Geometry check sheet. Reference: the model listing, model coordinates, mm. A direction names the side the tool comes from. Coordinates: 2 decimals unless noted, no trailing zeros. Write each loop counter-clockwise with the first axis right and the second up, starting at its lowest first coordinate (ties: lowest second). Pieces come first, ordered by that corner, then holes. Notation, with made-up numbers: (43, 47.25) -> (56, 47.25) arc R22 ccw to (56, 53.25) -> close; hole circle Ø6 at (-31, -38). An arc over 180 degrees is marked (long way). Use a Markdown table: item, result.
Autodesk Inventor part; units mm, degrees
ref_plane "YZ Plane" through (0, 0, 0) normal (1, 0, 0) x (0, 1, 0)
ref_plane "XZ Plane" through (0, 0, 0) normal (0, 1, 0) x (-1, 0, 0)
ref_plane "XY Plane" through (0, 0, 0) normal (0, 0, 1) x (1, 0, 0)
sketch "Sketch1" plane through (0, 0, 0) normal (1, 0, 0) x (0, 1, 0)
  line L0 (0, 0) -> (-25.4, 0)
  line L1 (-25.4, 0) -> (-25.4, -25.4)
  line L2 (-25.4, -25.4) -> (0, -25.4)
  line L3 (0, -25.4) -> (0, 0)
  line L4 (-3.175, -22.225) -> (-22.225, -22.225)
  line L5 (-22.225, -22.225) -> (-22.225, -3.175)
  line L6 (-22.225, -3.175) -> (-3.175, -3.175)
  line L7 (-3.175, -3.175) -> (-3.175, -22.225)
  dimension "d0" = 25.4
  dimension "d1" = 25.4
  dimension "d2" = 3.175
extrude "Extrusion1" add sketch "Sketch1" along normal blind 476.25
sketch "Sketch2" plane through (0, 0, 0) normal (0, 1, 0) x (1, 0, 0)
  line L0 (0, 3.175) -> (0, 22.225)
  line L1 (0, 12.7) -> (476.25, 12.7) construction
  line L2 (0, 25.4) -> (476.25, 25.4)
  line L3 (476.25, 25.4) -> (476.25, 0)
  point P0 (0, 0)
  point P1 (438.15, 12.7)
  point P2 (12.7, 12.7)
  point P3 (38.1, 12.7)
  point P4 (459.3336, 11.7602)
  dimension "d6" = 12.7
  dimension "d7" = 12.7
  dimension "d8" = 38.1
  dimension "d9" = 38.1
  dimension "d10" = 16.9164
  dimension "d11" = 13.6398
hole "Hole1" at (438.15, 0, -12.7) at (12.7, 0, -12.7) at (38.1, 0, -12.7) at (459.3336, 0, -11.7602) direction (0, -1, 0) diameter 6.35 end through all
properties part number "15102898-16-P-0307" material "Aluminum 6061"
Item 1: Mould release check, pull along Z, two halves, no side actions. Record for faces 1 (the flat face through (235, -3.175, -13)), 2 (the flat face through (235, -13, -25.4)), 3 (the flat face through (476.25, -2, -13)), 4 (the flat face through (235, -13, 0)): +Z half, -Z half, draft (parallel to the pull), parting line (faces both ways), or undercut.
Answer block:
| item | result |
|---|---|
| face 1 | undercut |
| face 2 | -Z half |
| face 3 | draft |
| face 4 | +Z half |
Item 2: Section check B-B on x = 296. Record the boundary of the cut face in (y, z) (3 decimals).
Answer block:
| item | result |
|---|---|
| outline | (-25.4, -25.4) -> (0, -25.4) -> (0, 0) -> (-25.4, 0) -> close; hole (-22.225, -22.225) -> (-3.175, -22.225) -> (-3.175, -3.175) -> (-22.225, -3.175) -> close |
Item 3: Thickness scan on L1, parallel to Y at x = 178, z = -20.5 (3 decimals); L2, parallel to Z at x = 38.1, y = -24.55 (3 decimals). Record the ranges inside material, lowest first. Write a range as [from, to].
Answer block:
| item | result |
|---|---|
| L1 | y = [-25.4, -22.225], [-3.175, 0] |
| L2 | z = [-25.4, -15.875], [-9.525, 0] |
Item 4: Section check A-A on y = -10.5. Record the boundary of the cut face in (x, z) (3 decimals).
Answer block:
| item | result |
|---|---|
| outline | (0, -25.4) -> (476.25, -25.4) -> (476.25, -22.225) -> (0, -22.225) -> close; (0, -3.175) -> (476.25, -3.175) -> (476.25, 0) -> (0, 0) -> close |
Item 5: Tool access check on faces 5 (the flat face through (235, -13, -3.175)), 6 (the flat face through (235, 0, -13)). Record the directions out of +Z, -Z, +X, -X, +Y, -Y that give a thin tool (end or side, any length) a straight path to the whole face; none if there is none.
Answer block:
| item | result |
|---|---|
| face 5 | +X, -X |
| face 6 | +Z, -Z, +X, -X, +Y |
